from build123d import *

# Parameters (mm, degrees)
SKETCH_1_W                     = 103.2
SKETCH_1_H                     = 20
EXTRUDE_1_DEPTH                = 39.7
SKETCH_2_W                     = 88.2
SKETCH_2_H                     = 33.7
CUT_EXTRUDE_1_DEPTH            = 17
EXTRUDE_START                  = -3
SKETCH_3_W                     = 26.5
SKETCH_3_H                     = 50
EXTRUDE_2_DEPTH                = 29
SKETCH_21_W                    = 20.5
SKETCH_21_H                    = 20.5
CUT_EXTRUDE_11_DEPTH           = 30.15
SKETCH_22_W                    = 20.2
SKETCH_22_H                    = 50
CUT_EXTRUDE_12_DEPTH           = 3.5
CUT_EXTRUDE_14_DEPTH           = 65.85
EXTRUDE_4_DEPTH                = 3
HOLE_WIZARD_M2_5_1_D           = 2.9
HOLE_WIZARD_M2_5_1_CSINK_D     = 2.95
HOLE_WIZARD_M2_5_1_CSINK_ANGLE = 90
HOLE_WIZARD_M5_2_D             = 5.5
HOLE_WIZARD_M5_2_CSINK_D       = 5.55
HOLE_WIZARD_M5_2_CSINK_ANGLE   = 90
CUT_EXTRUDE_19_DEPTH           = 51
SKETCH_36_W                    = 50
SKETCH_36_H                    = 46
CUT_EXTRUDE_20_DEPTH           = 51.6


with BuildPart() as part:
    # 草图1 → 凸台-拉伸1 (new body)
    with BuildSketch(Plane.XY):
        with Locations((-51.6, 10)):
            Rectangle(SKETCH_1_W, SKETCH_1_H)
    extrude(amount=EXTRUDE_1_DEPTH)

    # 草图2 → 切除-拉伸1 (cut)
    with BuildSketch(Plane(origin=(0, 20, 0), x_dir=(1, 0, 0), z_dir=(0, 1, 0))):
        with Locations((-51.6, -19.85)):
            Rectangle(SKETCH_2_W, SKETCH_2_H)
    extrude(amount=-CUT_EXTRUDE_1_DEPTH, mode=Mode.SUBTRACT)

    # 草图3 → 凸台-拉伸2 (add)
    with BuildSketch(Plane.XZ.offset(EXTRUDE_START)):
        with Locations((-51.6, 25)):
            Rectangle(SKETCH_3_W, SKETCH_3_H)
    extrude(amount=EXTRUDE_2_DEPTH)

    # 草图21 → 切除-拉伸11 (cut)
    with BuildSketch(Plane.XY.offset(50)):
        with Locations((-51.6, -9.25)):
            Rectangle(SKETCH_21_W, SKETCH_21_H)
    extrude(amount=-CUT_EXTRUDE_11_DEPTH, mode=Mode.SUBTRACT)

    # 草图22 → 切除-拉伸12 (cut)
    with BuildSketch(Plane.XZ.offset(26)):
        with Locations((-51.6, 25)):
            Rectangle(SKETCH_22_W, SKETCH_22_H)
    extrude(amount=-CUT_EXTRUDE_12_DEPTH, mode=Mode.SUBTRACT)

    # 草图24 → 切除-拉伸14 (cut, through all)
    with BuildSketch(Plane(origin=(-38.35, 0, 0), x_dir=(0, 0, -1), z_dir=(1, 0, 0))):
        Polygon((0, 0), (0, -26), (-19.85, -26), align=None)
    extrude(amount=-CUT_EXTRUDE_14_DEPTH, mode=Mode.SUBTRACT)

    # 草图25 → 凸台-拉伸4 (add)
    with BuildSketch(Plane.XZ):
        Polygon((-38.35, 39.7), (-38.35, 50), (0, 39.7), align=None)
        Polygon((-64.85, 39.7), (-103.2, 39.7), (-64.85, 50), align=None)
    extrude(amount=-EXTRUDE_4_DEPTH)

    # M2.5 间隙孔1 (through all)
    with Locations(Plane(origin=(0, 0, 0), x_dir=(-1, 0, 0), z_dir=(0, 0, -1))):
        with Locations((81.6, 9.75), (37.6, 9.75), (21.6, 9.75), (65.6, 9.75)):
            CounterSinkHole(HOLE_WIZARD_M2_5_1_D / 2, HOLE_WIZARD_M2_5_1_CSINK_D / 2, counter_sink_angle=HOLE_WIZARD_M2_5_1_CSINK_ANGLE)

    # M5 间隙孔2 (through all)
    with Locations(Plane(origin=(-38.35, 0, 0), x_dir=(0, 0, -1), z_dir=(1, 0, 0))):
        with Locations((-40.85, -9.25), (-25.85, -9.25)):
            CounterSinkHole(HOLE_WIZARD_M5_2_D / 2, HOLE_WIZARD_M5_2_CSINK_D / 2, counter_sink_angle=HOLE_WIZARD_M5_2_CSINK_ANGLE)

    # 草图35 → 切除-拉伸19 (cut, through all)
    with BuildSketch(Plane(origin=(0, 0, 0), x_dir=(-1, 0, 0), z_dir=(0, 0, -1))):
        Polygon((103.2, 20), (81.6, 20), (103.2, 9.75), align=None)
        Polygon((0, 20), (0, 9.75), (21.6, 20), align=None)
        Polygon((65.6, 20), (51.6, 15), (37.6, 20), align=None)
    extrude(amount=-CUT_EXTRUDE_19_DEPTH, mode=Mode.SUBTRACT)

    # 草图36 → 切除-拉伸20 (cut)
    with BuildSketch(Plane.ZY.offset(51.6)):
        with Locations((25, -3)):
            Rectangle(SKETCH_36_W, SKETCH_36_H)
    extrude(amount=-CUT_EXTRUDE_20_DEPTH, mode=Mode.SUBTRACT)


solid = part.part
Geometry: final body of the model. Coordinates: model frame, mm. A direction names the side the tool comes from. Round coordinates to 2 decimals unless told otherwise and drop trailing zeros. Order: outer loops, then holes, each group sorted by start corner. A loop starts at its lowest first (then second) coordinate and runs counter-clockwise, first axis right, second up.
Q1. Material intervals for probe 1 along Y at (x, z) = (-63.5, 25.85); probe 2 along Y at (x, z) = (-81.6, 1.05); probe 3 along Z at (x, y) = (-84.5, 11.5), sorted ascending.
Result sheet:
probe 1: y = -26 to -12, -6.5 to 3
probe 2: y = 0 to 8.3, 11.2 to 20
probe 3: z = 0 to 3, 36.7 to 39.7
Q2. Section C-C, the plane y = 4. Output: boundary loops of the cut face in (x, z).
Result sheet:
outline: (-103.2, 0) - (-51.6, 0) - (-51.6, 3) - (-95.7, 3) - (-95.7, 36.7) - (-51.6, 36.7) - (-51.6, 39.7) - (-103.2, 39.7) - close
Q3. Access query for faces 1 (the face through (-61.85, -9, 35)), 2 (the face through (-61.7, -24, 33)), 3 (the face through (-74, 12, 36.7)). Directions: +Z, -Z, +X, -X, +Y, -Y. A direction counts if a zero-diameter tool reaches every point of the face in a straight line with its end or side. Return the directions, or none.
Result sheet:
face 1: +Z, +X
face 2: +Z, -Z, +X, -Y
face 3: +X, +Y
Q4. Mould query, pull axis X, two halves, no side actions, for faces 4 (the face through (-66.75, 8.87, 1.53)), 5 (the face through (-97.05, 12.67, 19.57)), 6 (the face through (-57, -19.5, 35)). Classes: released by +X, released by -X, zero draft, split by the parting line, or undercut.
Result sheet:
face 4: undercut
face 5: released by -X
face 6: zero draft
Q5. Pin query (flat end, axial travel): pin 1 (1 mm diameter, centred on y = -1, z = 33, fed in from -X); pin 2 (5 mm diameter, centred on x = -57, y = -5.5, fed in from +Z); pin 3 (5 mm diameter, centred on y = 8, z = 13, fed in from +X). Return the tip coordinate at first contact, or that it passes through.
Result sheet:
pin 1: stops at x = -64.85
pin 2: stops at z = 19.85
pin 3: stops at x = -95.7
Q6. Section B-B, the plane y = -9.25. Output: boundary loops of the cut face in (x, z).
Result sheet:
outline: (-64.85, 7.06) - (-51.6, 7.06) - (-51.6, 19.85) - (-61.85, 19.85) - (-61.85, 23.1) - (-64.85, 23.1) - close; (-64.85, 28.6) - (-61.85, 28.6) - (-61.85, 38.1) - (-64.85, 38.1) - close; (-64.85, 43.6) - (-61.85, 43.6) - (-61.85, 50) - (-64.85, 50) - close
Q7. Section A-A, the plane z = 25.85. Output: boundary loops of the cut face in (x, y).
Result sheet:
outline: (-103.2, 0) - (-64.85, 0) - (-64.85, -6.5) - (-61.85, -6.5) - (-61.85, 1) - (-51.6, 1) - (-51.6, 3) - (-95.7, 3) - (-95.7, 13.31) - (-103.2, 9.75) - close; (-64.85, -26) - (-61.7, -26) - (-61.7, -22.5) - (-51.6, -22.5) - (-51.6, -19.5) - (-61.85, -19.5) - (-61.85, -12) - (-64.85, -12) - close
Q8. Section D-D, the plane x = -90. Output: boundary loops of the cut face in (y, z), and give its area (3 significant figures).
Result sheet:
outline: (0, 0) - (16.01, 0) - (16.01, 3) - (3, 3) - (3, 36.7) - (16.01, 36.7) - (16.01, 39.7) - (3, 39.7) - (3, 43.25) - (0, 43.25) - close
area: 208 mm2
